Can you work these out from the model? Positions are in its coordinate system, mm. A direction names the side the tool comes from. Round coordinates to 2 decimals unless told otherwise and drop trailing zeros. Order: outer loops, then holes, each group sorted by start corner. A loop starts at its lowest first (then second) coordinate and runs counter-clockwise, first axis right, second up. Notation, with made-up numbers: M 76.25,70.5 L 114.25,70.5 A26 ccw 114.25,97.5 Z; hole C 9.25,1.5 d4. An arc over 180 degrees is marked long. Answer as a JSON object with one key per item and string values. Group by question number.
```python
from build123d import *

# Parameters (mm, degrees)
F0_W     = 381
F0_H     = 381
F1_DEPTH = 25.4
F2_W     = 101.6
F2_H     = 101.6
F3_DEPTH = 12.7
F4_R     = 10
F5_R     = 15.875
F6_DEPTH = 50


with BuildPart() as f1:
    # F0 (on Top) → F1 (new body)
    with BuildSketch(Plane.XY):
        Rectangle(F0_W, F0_H)
    extrude(amount=F1_DEPTH)

    # F2 (on face) → F3 (cut)
    with BuildSketch(Plane.XY.offset(25.4)):
        Rectangle(F2_W, F2_H)
    extrude(amount=-F3_DEPTH, mode=Mode.SUBTRACT)

    # F4
    f4_edges = [f1.edges().sort_by_distance(p)[0] for p in [
        (50.8, 50.8, 19.05),
        (-50.8, 50.8, 19.05),
        (-50.8, -50.8, 19.05),
        (50.8, -50.8, 19.05),
    ]]
    fillet(f4_edges, radius=F4_R)

    # F5 (on face) → F6 (cut)
    with BuildSketch(Plane.XY.offset(25.4)):
        with Locations((-152.4, -152.4)):
            Circle(F5_R)
        with Locations((-152.4, 152.4)):
            Circle(F5_R)
        with Locations((152.4, -152.4)):
            Circle(F5_R)
        with Locations((152.4, 152.4)):
            Circle(F5_R)
    extrude(amount=-F6_DEPTH, mode=Mode.SUBTRACT)


solid = f1.part
```
1) I need wall thicknesses on line 1 along Y through (x, z) = (152.4, 8.25) (3 decimals); line 2 along X through (y, z) = (-146, 13); line 3 along X through (y, z) = (-34, 23). Which ranges of each line are inside material? Lowest first, please.
2) If we section it at A-A on x = -152.4: Write out the boundary of the cut face in (y, z) (3 decimals).
3) If we section it at D-D on x = -10: Write out the boundary of the cut face in (y, z), plus the area to 3 significant figures.
4) Which directions (+Z, -Z, +X, -X, +Y, -Y) give clear straight access to the entire face, cutting with the end or side of a thin tool? Please do faces 4 (the face through (-1, 1, 12.7)), 5 (the face through (150.33, 168.14, 12.88)).
5) We'd pull the mould along Y, two halves only. Please class faces 1 (the face through (-190.5, -3, 13)), 2 (the face through (-3, -190.5, 13)), 3 (the face through (47.95, 47.79, 18.96)): +Y half, -Y half, draft (parallel to the pull), parting line (faces both ways), or undercut.
6) If we section it at B-B on z = 19.5: Write out the boundary of the cut face in (x, y) (3 decimals).
Findings:
{
 "1": {"line 1": "y = -190.5 to -168.275, -136.525 to 136.525, 168.275 to 190.5", "line 2": "x = -190.5 to -166.93, -137.87 to 137.87, 166.93 to 190.5", "line 3": "x = -190.5 to -50.8, 50.8 to 190.5"},
 "2": {"outline": "M -190.5,0 L -168.275,0 L -168.275,25.4 L -190.5,25.4 Z; M -136.525,0 L 136.525,0 L 136.525,25.4 L -136.525,25.4 Z; M 168.275,0 L 190.5,0 L 190.5,25.4 L 168.275,25.4 Z"},
 "3": {"outline": "M -190.5,0 L 190.5,0 L 190.5,25.4 L 50.8,25.4 L 50.8,12.7 L -50.8,12.7 L -50.8,25.4 L -190.5,25.4 Z", "area": "8,390 mm^2"},
 "4": {"face 4": "+Z", "face 5": "+Z, -Z"},
 "5": {"face 1": "draft", "face 2": "-Y half", "face 3": "undercut"},
 "6": {"outline": "M -190.5,-190.5 L 190.5,-190.5 L 190.5,190.5 L -190.5,190.5 Z; hole C -152.4,-152.4 d31.75; hole C -152.4,152.4 d31.75; hole M -50.8,-40.8 A10 ccw -40.8,-50.8 L 40.8,-50.8 A10 ccw 50.8,-40.8 L 50.8,40.8 A10 ccw 40.8,50.8 L -40.8,50.8 A10 ccw -50.8,40.8 Z; hole C 152.4,-152.4 d31.75; hole C 152.4,152.4 d31.75"}
}
